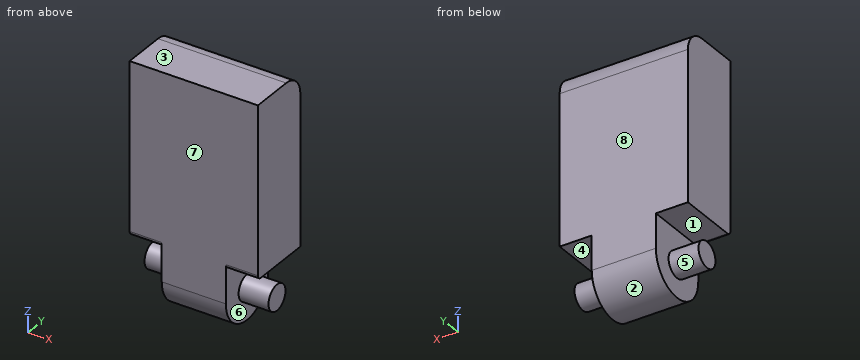
```python
from build123d import *

# Parameters (mm, degrees)
SKETCH_1_W      = 30
SKETCH_1_H      = 15
EXTRUDE_1_DEPTH = 40
EXTRUDE_3_DEPTH = 7.5
SKETCH_7_R      = 3
EXTRUDE_4_DEPTH = 7
FILLET_1_R      = 5
FILLET_2_R      = 1


with BuildPart() as part:
    # 草图1 → 凸台-拉伸1 (new body)
    with BuildSketch(Plane.XY):
        Rectangle(SKETCH_1_W, SKETCH_1_H)
    extrude(amount=EXTRUDE_1_DEPTH)

    # 草图6 → 凸台-拉伸3 (add, symmetric)
    with BuildSketch(Plane(origin=(0, 0, 0), x_dir=(0, 0, -1), z_dir=(1, 0, 0))):
        with BuildLine():
            Line((0, 7.5), (8, 7.5))
            ThreePointArc((8, 7.5), (15.5, 0), (8, -7.5))
            Line((8, -7.5), (0, -7.5))
            Line((0, -7.5), (0, 7.5))
        make_face()
    extrude(amount=EXTRUDE_3_DEPTH, both=True)

    # 草图7 → 凸台-拉伸4 (add)
    with BuildSketch(Plane(origin=(7.5, 0, 0), x_dir=(0, 0, -1), z_dir=(1, 0, 0))):
        with Locations(Location((8, 0, 0), (0, 0, 180))):
            Circle(SKETCH_7_R)
    extrude_4 = extrude(amount=EXTRUDE_4_DEPTH)

    # 镜向2: 凸台-拉伸4 across plane
    add(extrude_4.mirror(Plane(origin=(0, 0, 0), x_dir=(0, 0, 1), z_dir=(1, 0, 0))))

    # 圆角1
    fillet_1_edges = [part.edges().sort_by_distance(p)[0] for p in [
        (0, 7.5, 40),
    ]]
    fillet(fillet_1_edges, radius=FILLET_1_R)

    # 圆角2
    fillet_2_edges = [part.edges().sort_by_distance(p)[0] for p in [
        (11.25, -7.5, 0),
        (-11.25, -7.5, 0),
    ]]
    fillet(fillet_2_edges, radius=FILLET_2_R)


solid = part.part
```
Input: part model. Units: mm. Frame: model coordinates. Face numbers are marked on the shaded views. A direction names the side the tool comes from. Coordinates: 2 decimals unless noted, no trailing zeros. Write each loop counter-clockwise with the first axis right and the second up, starting at its lowest first coordinate (ties: lowest second). Pieces come first, ordered by that corner, then holes.
1) Set-up query: the marked faces 4, 5, 6, 7 and 8. Return all of +Z, -Z, +X, -X, +Y, -Y with unobstructed straight access to the full face (end or side cutting, diameter ignored); none if empty.
2) Section B-B on y = 0. Output: boundary loops of the cut face in (x, z), and give its area (3 significant figures).
3) Section A-A on x = -12.5. Output: boundary loops of the cut face in (y, z).
4) Mould query, pull axis Z, two halves, no side actions, for the marked faces 1, 2 and 3. Classes: pulls with the +Z half, pulls with the -Z half, needs draft (parallel to the pull), parting line crosses it, or undercut.
5) Material intervals for line 1 along X through (y, z) = (-1.25, -0.5); line 2 along Z through (x, y) = (9.75, -1.25); line 3 along Z through (x, y) = (13.5, -2.5), sorted ascending.
6) Pin query (flat end, axial travel): pin 1 Ø4.5 at (y, z) = (2.5, -9) entering from -X; pin 2 Ø6.5 at (y, z) = (0.5, -8) entering from +X; pin 3 Ø6 at (x, y) = (-12, 1.5) entering from -Z. Return the tip coordinate at first contact, or that it passes through.
Check result:
1. face 4: +X, +Y, -Y
1. face 5: -X
1. face 6: +X
1. face 7: +Z, -Z, +X, -X, -Y
1. face 8: +Z, -Z, +X, -X, +Y
2. outline: (-15, 0) - (-7.5, 0) - (-7.5, -5) - (-14.5, -5) - (-14.5, -11) - (-7.5, -11) - (-7.5, -15.5) - (7.5, -15.5) - (7.5, -11) - (14.5, -11) - (14.5, -5) - (7.5, -5) - (7.5, 0) - (15, 0) - (15, 40) - (-15, 40) - close
2. area: 1,520 mm2
3. outline: (-7.5, 1) arc R1 ccw to (-6.5, 0) - (7.5, 0) - (7.5, 35) arc R5 ccw to (2.5, 40) - (-7.5, 40) - close; circle Ø6 at (0, -8)
4. face 1: undercut
4. face 2: pulls with the -Z half
4. face 3: pulls with the +Z half
5. line 1: x = -7.5 to 7.5
5. line 2: z = -10.73 to -5.27, 0 to 40
5. line 3: z = -9.66 to -6.34, 0 to 40
6. pin 1: stops at x = -14.5
6. pin 2: stops at x = 14.5
6. pin 3: stops at z = -11
